Check sheet for the modelled part. Datum: model origin and axes. Units: mm. Coordinates: 2 decimals unless noted, no trailing zeros. Answer as CSV lines item,"result". Start each with the question number.
Q1. Sectioned sample at A-A, the plane z = -332.5. Count the separate pieces of the cut face and the enclosed holes in it, then the cut area to 3 significant figures.
Q2. Depth check by flat-ended pin: pin 1 Ø2.5 at (y, z) = (11.5, -463) entering from +X; pin 2 Ø1.9 at (x, z) = (8, -246) entering from +Y; pin 3 Ø5.5 at (x, z) = (10, -328.5) entering from +Y; pin 4 Ø1.9 at (x, z) = (-5.5, -454) entering from -Y. Enter the tip coordinate at first touch or a pass-through.
Q3. Thickness scan on line 1 along X through (y, z) = (10.5, -425.5); line 2 along Y through (x, z) = (17, -382); line 3 along Y through (x, z) = (-10, -616). Record the ranges inside material, lowest first. Write a range as from..to.
from build123d import *

# Parameters (mm, degrees)
SKETCH2_R           = 2
BOSS_EXTRUDE1_DEPTH = 800


with BuildPart() as part:
    # Sketch2 → Boss-Extrude1 (new body)
    with BuildSketch(Plane.XY):
        Polygon((-13.9, -12.839339828), (-13.9, -10.519615242), (-13.6, -10), (-13.9, -9.480384758), (-13.9, -7.160660172), (-16.56, -4.500660172), (-18.2, -4.500660172), (-18.2, -6.900379336), (-20, -5.39), (-20, 5.39), (-18.2, 6.900379336), (-18.2, 4.500660172), (-16.56, 4.500660172), (-13.9, 7.160660172), (-13.9, 9.480384758), (-13.6, 10), (-13.9, 10.519615242), (-13.9, 12.839339828), (-16.560660172, 15.5), (-18.2, 15.5), (-18.2, 13.099620664), (-20, 14.61), (-20, 20), (-14.61, 20), (-13.099620664, 18.2), (-15.5, 18.2), (-15.5, 16.560660172), (-12.839339828, 13.9), (-10.519615242, 13.9), (-10, 13.6), (-9.480384758, 13.9), (-7.160660172, 13.9), (-4.500660172, 16.56), (-4.500660172, 18.2), (-6.900379336, 18.2), (-5.39, 20), (5.39, 20), (6.900379336, 18.2), (4.500660172, 18.2), (4.500660172, 16.56), (7.160660172, 13.9), (9.480384758, 13.9), (10, 13.6), (10.519615242, 13.9), (12.839339828, 13.9), (15.5, 16.560660172), (15.5, 18.2), (13.099620664, 18.2), (14.61, 20), (20, 20), (20, 14.61), (18.2, 13.099620664), (18.2, 15.5), (16.560660172, 15.5), (13.9, 12.839339828), (13.9, 10.519615242), (13.6, 10), (13.9, 9.480384758), (13.9, 7.160660172), (16.56, 4.500660172), (18.2, 4.500660172), (18.2, 6.900379336), (20, 5.39), (20, -5.39), (18.2, -6.900379336), (18.2, -4.500660172), (16.56, -4.500660172), (13.9, -7.160660172), (13.9, -9.480384758), (13.6, -10), (13.9, -10.519615242), (13.9, -12.839339828), (16.560660172, -15.5), (18.2, -15.5), (18.2, -13.099620664), (20, -14.61), (20, -20), (14.61, -20), (13.099620664, -18.2), (15.5, -18.2), (15.5, -16.560660172), (12.839339828, -13.9), (10.519615242, -13.9), (10, -13.6), (9.480384758, -13.9), (7.160660172, -13.9), (4.500660172, -16.56), (4.500660172, -18.2), (6.900379336, -18.2), (5.39, -20), (-5.39, -20), (-6.900379336, -18.2), (-4.500660172, -18.2), (-4.500660172, -16.56), (-7.160660172, -13.9), (-9.480384758, -13.9), (-10, -13.6), (-10.519615242, -13.9), (-12.839339828, -13.9), (-15.5, -16.560660172), (-15.5, -18.2), (-13.099620664, -18.2), (-14.61, -20), (-20, -20), (-20, -14.61), (-18.2, -13.099620664), (-18.2, -15.5), (-16.560660172, -15.5), align=None)
        with Locations((-10, -10)):
            Circle(SKETCH2_R, mode=Mode.SUBTRACT)
        with Locations((10, -10)):
            Circle(SKETCH2_R, mode=Mode.SUBTRACT)
        with Locations((10, 10)):
            Circle(SKETCH2_R, mode=Mode.SUBTRACT)
        with Locations((-10, 10)):
            Circle(SKETCH2_R, mode=Mode.SUBTRACT)
        Polygon((-12.839339828, -6.1), (-6.1, -6.1), (-6.1, -12.839339828), (-2.379339828, -16.56), (-2.379339828, -18.2), (2.379339828, -18.2), (2.379339828, -16.56), (6.1, -12.839339828), (6.1, -6.1), (12.839339828, -6.1), (16.56, -2.379339828), (18.2, -2.379339828), (18.2, 2.379339828), (16.56, 2.379339828), (12.839339828, 6.1), (6.1, 6.1), (6.1, 12.839339828), (2.379339828, 16.56), (2.379339828, 18.2), (-2.379339828, 18.2), (-2.379339828, 16.56), (-6.1, 12.839339828), (-6.1, 6.1), (-12.839339828, 6.1), (-16.56, 2.379339828), (-18.2, 2.379339828), (-18.2, -2.379339828), (-16.56, -2.379339828), align=None, mode=Mode.SUBTRACT)
    extrude(amount=-BOSS_EXTRUDE1_DEPTH)


solid = part.part
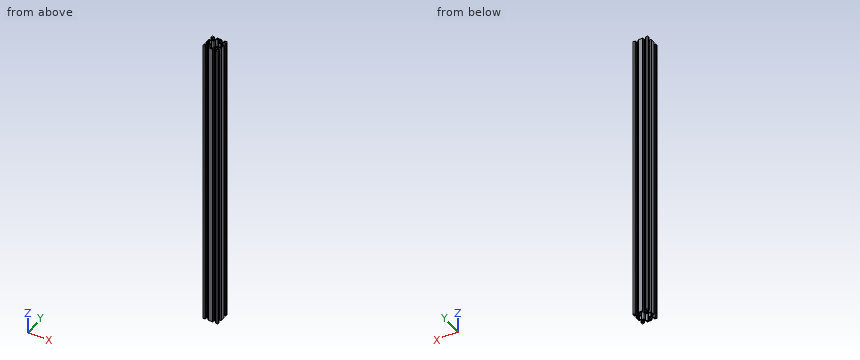
Output:
1,separate pieces,"1"
1,enclosed holes,"5"
1,area,"481 mm^2"
2,pin 1,"stops at x = 13.9"
2,pin 2,"stops at y = 14.01"
2,pin 3,"stops at y = 13.9"
2,pin 4,"stops at y = -20"
3,line 1,"x = -13.89..-11.94, -8.06..-6.1, 6.1..8.06, 11.94..13.89"
3,line 2,"y = -20..-15.5, -4.5..-2.38, 2.38..4.5, 15.5..20"
3,line 3,"y = -13.6..-12, -8..-6.1, 6.1..8, 12..13.6"
